```python
from build123d import *

# Parameters (mm, degrees)
CROQUIS1_R              = 1.2
SALIENTE_EXTRUIR1_DEPTH = 12.7


with BuildPart() as part:
    # Croquis1 → Saliente-Extruir1 (new, symmetric)
    with BuildSketch(Plane.XY):
        Circle(CROQUIS1_R)
    extrude(amount=SALIENTE_EXTRUIR1_DEPTH, both=True)

    # Croquis4 → Revolución1 (revolve)
    with BuildSketch(Plane(origin=(0, 0, 0), x_dir=(1, 0, 0), z_dir=(0, 1, 0))):
        with BuildLine():
            Line((0, -13.5), (0, -12.7))
            Line((0, -12.7), (-1.5, -12.7))
            ThreePointArc((-1.5, -12.7), (-0.85, -13.2875), (0, -13.5))
        make_face()
    revoluci_n1 = revolve(axis=Axis((0, 0, 13.5), (0, 0, -1)))

    # Simetría1: Revolución1 across plane
    add(revoluci_n1.mirror(Plane.XY))


solid = part.part
```
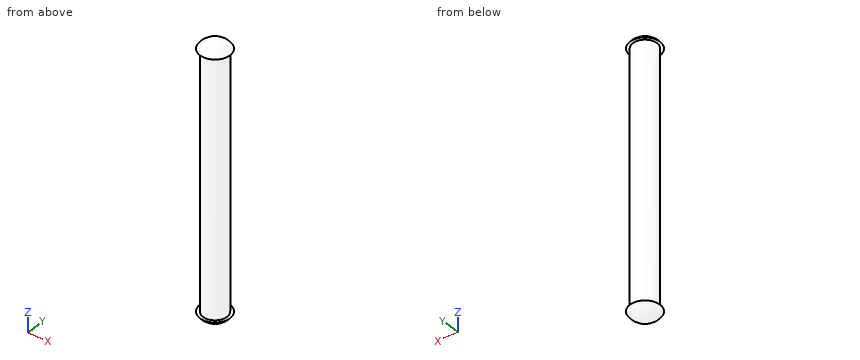
Read the model definition and answer for the solid it produces. Units are mm, in the model's axes. Coordinates: 2 decimals unless noted, no trailing zeros. Loops run counter-clockwise (first coordinate to the right, second up) from the corner with the lowest first, then second, coordinate; pieces in that order, holes last.
(1) The part is cut by section C-C (z = -6.5). Determine the outline of the cut face in (x, y), and give its area (3 significant figures).
Solution:
outline: circle Ø2.4 at (0, 0)
area: 4.52 mm2
(2) Consider line 1 along Z through (x, y) = (1.35, -0.1); line 2 along Y through (x, z) = (-0.1, -2). Determine where each line is inside the solid, lowest interval first.
Solution:
line 1: z = -12.89 to -12.7, 12.7 to 12.89
line 2: y = -1.2 to 1.2
(3) The part is cut by section A-A (y = 0). Determine the outline of the cut face in (x, z).
Solution:
outline: (-1.5, -12.7) arc R1.81 ccw to (1.5, -12.7) - (1.2, -12.7) - (1.2, 12.7) - (1.5, 12.7) arc R1.81 ccw to (-1.5, 12.7) - (-1.2, 12.7) - (-1.2, -12.7) - close
(4) Flat-ended cylindrical pins translate along their axes: pin 1 Ø1.5 at (x, z) = (-0.5, -3.5) entering from -Y; pin 2 Ø1 at (x, y) = (-0.5, 0.5) entering from +Z. Find the tip coordinate at first contact, or state that the pin passes through.
Solution:
pin 1: stops at y = -1.2
pin 2: stops at z = 13.49
